```python
from build123d import *

# Parameters (mm, degrees)
CUT_EXTRUDE1_DEPTH     = 2
CUT_SWEEP6_PITCH       = 1.62
CUT_SWEEP6_HEIGHT      = 40
CUT_SWEEP6_RADIUS      = 3.5
CUT_SWEEP6_START_ANGLE = -45


with BuildPart() as part:
    # Sketch1 → Revolve1 (revolve)
    with BuildSketch(Plane(origin=(0, 0, 0), x_dir=(1, 0, 0), z_dir=(0, 1, 0))):
        Polygon((0, 0), (0, 5), (0.2, 5), (2, 3.5), (8.466666667, 3.5), (10, 2.35), (50, 2.35), (50, 0), align=None)
    revolve(axis=Axis((50, 0, 0), (-1, 0, 0)))

    # Sketch2 → Cut-Extrude1 (cut)
    with BuildSketch(Plane.ZY):
        Polygon((1.987284991, 1.176448765), (-0.025192021, 2.30926367), (-2.012477012, 1.132814905), (-1.987284991, -1.176448765), (0.025192021, -2.30926367), (2.012477012, -1.132814905), align=None)
    extrude(amount=-CUT_EXTRUDE1_DEPTH, mode=Mode.SUBTRACT)

    # Cut-Sweep6: sweep along a helix
    with BuildLine() as cut_sweep6_path:
        add(Helix(CUT_SWEEP6_PITCH, CUT_SWEEP6_HEIGHT, CUT_SWEEP6_RADIUS, center=(50, 0, 0), direction=(-1, 0, 0), mode=Mode.PRIVATE).rotate(Axis((50, 0, 0), (-1, 0, 0)), CUT_SWEEP6_START_ANGLE))
    # Sketch6 → Cut-Sweep6 (sweep, cut)
    with BuildSketch(Plane(origin=(0, 0, 0), x_dir=(1, 0, 0), z_dir=(0, 1, 0))):
        Polygon((50, 2.474873734), (49.595000005, 2.474873734), (49.797500002, 3.500000136), align=None)
    sweep(path=cut_sweep6_path.line, is_frenet=True, mode=Mode.SUBTRACT)


solid = part.part
```
Input: part model. Units: mm. Frame: model coordinates. A direction names the side the tool comes from. Give positions to 0.01 mm unless a question says otherwise; leave off trailing zeros. Loops run counter-clockwise (first coordinate to the right, second up) from the corner with the lowest first, then second, coordinate; pieces in that order, holes last.
1) Section query A-A on x = 42. Return the cut outline in (y, z).
A:
outline: circle Ø4.7 at (0, 0)
2) Mould query, pull axis Z, two halves, no side actions, for faces 4 (the cylindrical face through (30.28, 2.294, 0.509)), 5 (the flat face through (50, 0, 0)), 6 (the flat face through (0.99, 1.73, -1)). Classes: released by +Z, released by -Z, zero draft, split by the parting line, or undercut.
A:
face 4: split by the parting line
face 5: zero draft
face 6: undercut
3) Section query B-B on y = 0. Return the cut outline in (x, z), and give its area (3 significant figures).
A:
outline: (0, -5) - (0.2, -5) - (2, -3.5) - (8.47, -3.5) - (10, -2.35) - (50, -2.35) - (50, 2.35) - (10, 2.35) - (8.47, 3.5) - (2, 3.5) - (0.2, 5) - (0, 5) - (0, 2) - (2, 2) - (2, -2) - (0, -2) - close
area: 252 mm2
4) Contact query for flat-ended pins moving along their axis: pin 1 (3 mm diameter, centred on x = 13, z = 3, fed in from +Y); pin 2 (4 mm diameter, centred on x = 6.5, z = 0.5, fed in from -Y); pin 3 (5 mm diameter, centred on x = 13.5, z = -3, fed in from +Y). Output: stop coordinate, or through.
A:
pin 1: stops at y = 1.81
pin 2: stops at y = -3.5
pin 3: stops at y = 2.3
5) Line query: L1, parallel to X at y = 0, z = -0.25; L2, parallel to Y at x = 3.5, z = -0.25; L3, parallel to Z at x = 29, y = 1.25. Output: solid intervals per line, ascending.
A:
L1: x = 2 to 50
L2: y = -3.49 to 3.49
L3: z = -1.99 to 1.99
6) Reachability of faces 1 (the cylindrical face through (5.279, 1.341, -3.233)), 2 (the flat face through (0, -0.1, 2.2)), 3 (the flat face through (0.99, -1.73, -1)) from +Z, -Z, +X, -X, +Y, -Y: full face, straight path, thin tool, end or side. Return the list, or none.
A:
face 1: +X
face 2: +Z, -Z, -X, +Y, -Y
face 3: -X
7) Section query C-C on x = 5.5. Return the cut outline in (y, z), and give its area (3 significant figures).
A:
outline: circle Ø7 at (0, 0)
area: 38.5 mm2
